Verification items for the finished model (mm, model axes). Give positions to 0.01 mm unless a question says otherwise; leave off trailing zeros. Write each loop counter-clockwise with the first axis right and the second up, starting at its lowest first coordinate (ties: lowest second). Pieces come first, ordered by that corner, then holes. Notation, with made-up numbers: (41, -8.5) -> (79, -8.5) arc R29 ccw to (79, 21.5) -> close; hole circle Ø9 at (61.25, 4). An arc over 180 degrees is marked (long way). Answer as CSV lines item,"result".
```python
from build123d import *

# Parameters (mm, degrees)
SKETCH_1_R          = 12.5
EXTRUDE_1_DEPTH     = 257
CUT_EXTRUDE_1_DEPTH = 0.975


with BuildPart() as part:
    # 草图1 → 凸台-拉伸1 (new body)
    with BuildSketch(Plane.XY):
        Circle(SKETCH_1_R)
    extrude(amount=EXTRUDE_1_DEPTH)

    # 草图6 → 切除-拉伸1 (cut, symmetric)
    with BuildSketch(Plane(origin=(0, 12, 0), x_dir=(1, 0, 0), z_dir=(0, 1, 0))):
        with BuildLine():
            Line((-4, -29.5), (-4, -25.5))
            ThreePointArc((-4, -25.5), (0, -21.5), (4, -25.5))
            Line((4, -25.5), (4, -29.5))
            ThreePointArc((4, -29.5), (0, -33.5), (-4, -29.5))
        make_face()
        with BuildLine():
            Line((-4, -126.5), (-4, -130.5))
            ThreePointArc((-4, -130.5), (0, -134.5), (4, -130.5))
            Line((4, -130.5), (4, -126.5))
            ThreePointArc((4, -126.5), (0, -122.5), (-4, -126.5))
        make_face()
    cut_extrude_1 = extrude(amount=CUT_EXTRUDE_1_DEPTH, both=True, mode=Mode.SUBTRACT)

    # 镜向1: 切除-拉伸1 across plane
    add(cut_extrude_1.mirror(Plane(origin=(0, 0, 128.5), x_dir=(1, 0, 0), z_dir=(0, 0, -1))), mode=Mode.SUBTRACT)


solid = part.part
```
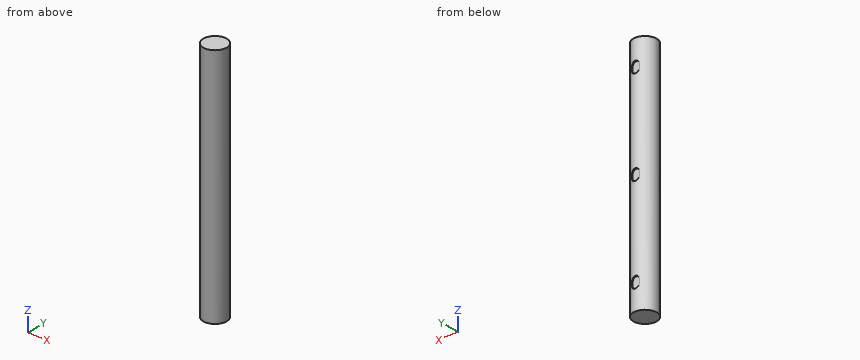
1) Depth check by flat-ended pin: pin 1 (4 mm diameter, centred on x = 1, z = 126, fed in from +Y) (3 decimals); pin 2 (0.9 mm diameter, centred on y = 11.5, z = 229, fed in from +X); pin 3 (4 mm diameter, centred on y = -9, z = 112.5, fed in from +X). Enter the tip coordinate at first touch or a pass-through.
Reported:
pin 1,"y = 11.025"
pin 2,"x = 5.84"
pin 3,"x = 10.36"
2) Section check B-B (z = 163.5). Record the boundary of the cut face in (x, y), and give its area (3 significant figures).
Reported:
outline,"circle Ø25 at (0, 0)"
area,"491 mm²"
3) Section check C-C (y = 6.25). Record the boundary of the cut face in (x, z).
Reported:
outline,"(-10.83, 0) -> (10.83, 0) -> (10.83, 257) -> (-10.83, 257) -> close"
4) Section check A-A (x = -1.75). Record the boundary of the cut face in (y, z) (3 decimals).
Reported:
outline,"(-12.377, 0) -> (12.377, 0) -> (12.377, 21.903) -> (11.025, 21.903) -> (11.025, 33.097) -> (12.377, 33.097) -> (12.377, 122.903) -> (11.025, 122.903) -> (11.025, 134.097) -> (12.377, 134.097) -> (12.377, 223.903) -> (11.025, 223.903) -> (11.025, 235.097) -> (12.377, 235.097) -> (12.377, 257) -> (-12.377, 257) -> close"
5) Section check D-D (x = 7.5). Record the boundary of the cut face in (y, z), and give its area (3 significant figures).
Reported:
outline,"(-10, 0) -> (10, 0) -> (10, 257) -> (-10, 257) -> close"
area,"5,140 mm²"
6) Scan lines: line 1 along Y through (x, z) = (0.5, 105.5); line 2 along Y through (x, z) = (-5.5, 215); line 3 along X through (y, z) = (-4.75, 69). Record each from-to range of solid material in increasing order.
Reported:
line 1,"-12.49 to 12.49"
line 2,"-11.22 to 11.22"
line 3,"-11.56 to 11.56"
